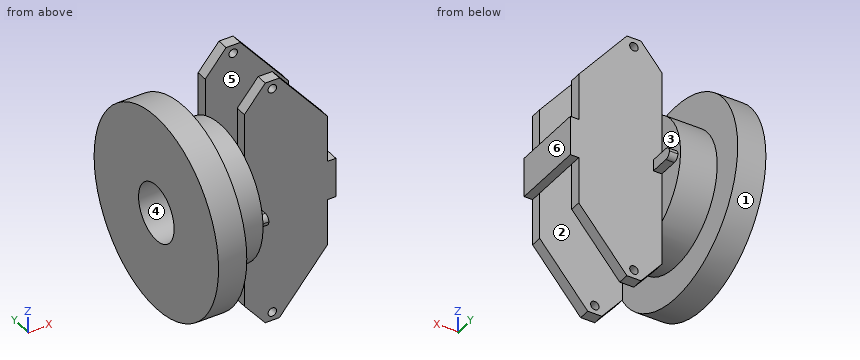
```python
from build123d import *

# Parameters (mm, degrees)
SKETCH1_R               = 35
BOSS_EXTRUDE1_DEPTH     = 10
SKETCH2_R               = 23.5
BOSS_EXTRUDE2_DEPTH     = 13
BOSS_EXTRUDE3_DEPTH     = 4
SKETCH5_R               = 1.5
CUT_EXTRUDE1_DEPTH      = 4
MIRROR3_COPY_1_SKETCH_R = 1.5
MIRROR3_COPY_1_DEPTH    = 4
BOSS_EXTRUDE4_DEPTH     = 3
FILLET1_R               = 2
FILLET1_OF_MIRROR5_R    = 2
SKETCH8_W               = 14
SKETCH8_H               = 26
BOSS_EXTRUDE5_DEPTH     = 3
SKETCH9_R               = 10
CUT_EXTRUDE2_DEPTH      = 10


with BuildPart() as part:
    # Sketch1 → Boss-Extrude1 (new body)
    with BuildSketch(Plane(origin=(0, 0, 0), x_dir=(0, 0, -1), z_dir=(1, 0, 0))):
        Circle(SKETCH1_R)
    extrude(amount=BOSS_EXTRUDE1_DEPTH)

    # Sketch2 → Boss-Extrude2 (add)
    with BuildSketch(Plane(origin=(10, 0, 0), x_dir=(0, 0, -1), z_dir=(1, 0, 0))):
        with Locations(Location((0, 0, 0), (0, 0, 180))):
            Circle(SKETCH2_R)
    extrude(amount=BOSS_EXTRUDE2_DEPTH)

    # Sketch3 → Boss-Extrude3 (add)
    with BuildSketch(Plane(origin=(0, 13, 0), x_dir=(1, 0, 0), z_dir=(0, 1, 0))):
        Polygon((23, 35), (23, -35), (30.392057511, -43.809511096), (35.392057511, -43.809511096), (52.421803319, -23.514250349), (52.421803319, 0), (52.421803319, 23.514250349), (35.392057511, 43.809511096), (30.392057511, 43.809511096), align=None)
    boss_extrude3 = extrude(amount=-BOSS_EXTRUDE3_DEPTH)

    # Sketch5 → Cut-Extrude1 (cut)
    with BuildSketch(Plane(origin=(0, 13, 0), x_dir=(1, 0, 0), z_dir=(0, 1, 0))):
        with Locations(Location((32.892057511, -40.809511096, 0), (0, 0, 270))):
            Circle(SKETCH5_R)
    cut_extrude1 = extrude(amount=-CUT_EXTRUDE1_DEPTH, mode=Mode.SUBTRACT)

    # Mirror2: Cut-Extrude1 across plane
    add(cut_extrude1.mirror(Plane.XY), mode=Mode.SUBTRACT)

    # Mirror3: Boss-Extrude3, Cut-Extrude1 across plane
    add(boss_extrude3.mirror(Plane.ZX))
    add(cut_extrude1.mirror(Plane.ZX), mode=Mode.SUBTRACT)

    # Mirror3 copy 1 sketch → Mirror3 copy 1 (cut)
    with BuildSketch(Plane.XZ.offset(13)):
        with Locations(Location((32.892057511, -40.809511096, 0), (0, 0, 270))):
            Circle(MIRROR3_COPY_1_SKETCH_R)
    extrude(amount=-MIRROR3_COPY_1_DEPTH, mode=Mode.SUBTRACT)

    # Sketch7 → Boss-Extrude4 (add)
    with BuildSketch(Plane(origin=(23, 0, 0), x_dir=(0, 0, -1), z_dir=(1, 0, 0))):
        Polygon((0, 22), (-2, 22), (-2, 13), (2, 13), (2, 22), align=None)
    boss_extrude4 = extrude(amount=BOSS_EXTRUDE4_DEPTH)

    # Fillet1
    fillet1_edges = [part.edges().sort_by_distance(p)[0] for p in [
        (24.5, 22, 2),
        (24.5, 22, -2),
    ]]
    fillet(fillet1_edges, radius=FILLET1_R - 0.0001)  # a hair under: the kernel refuses the full size

    # Mirror5: Boss-Extrude4 across plane
    add(boss_extrude4.mirror(Plane.ZX))

    # Fillet1 of Mirror5
    fillet1_of_mirror5_edges = [part.edges().sort_by_distance(p)[0] for p in [
        (24.5, -22, 2),
        (24.5, -22, -2),
    ]]
    fillet(fillet1_of_mirror5_edges, radius=FILLET1_OF_MIRROR5_R - 0.0001)  # a hair under: the kernel refuses the full size

    # Sketch8 → Boss-Extrude5 (add)
    with BuildSketch(Plane(origin=(52.421803319, 0, 0), x_dir=(0, 0, -1), z_dir=(1, 0, 0))):
        Rectangle(SKETCH8_W, SKETCH8_H)
    extrude(amount=BOSS_EXTRUDE5_DEPTH)

    # Sketch9 → Cut-Extrude2 (cut)
    with BuildSketch(Plane.ZY):
        Circle(SKETCH9_R)
    extrude(amount=-CUT_EXTRUDE2_DEPTH, mode=Mode.SUBTRACT)


solid = part.part
```
Here's how the part is built. I have some questions about the finished solid (model axes, mm). Face numbers are marked on the shaded views. A direction names the side the tool comes from. Coordinates: 2 decimals unless noted, no trailing zeros. Order: outer loops, then holes, each group sorted by start corner. A loop starts at its lowest first (then second) coordinate and runs counter-clockwise, first axis right, second up. Notation, with made-up numbers: (85, -36) -> (89, -36) arc R16 ccw to (89, -18) -> close; hole circle Ø9 at (-8, 23). An arc over 180 degrees is marked (long way). Return JSON: item names as keys, results as strings.
1) I'm going to push flat-ended pins straight in: P1, Ø4.5, axis at y = 11.5, z = 15.5, coming from the +X side; P2, Ø3, axis at x = 41.5, z = -17.5, coming from the +Y side; P3, Ø4.5, axis at y = 10, z = 27.5, coming from the -X side; P4, Ø2.5, axis at x = 24.5, y = 15, coming from the +Z side. Where does each tip first touch, or does it pass through?
Conclusion:
{"P1": "stops at x = 52.42", "P2": "stops at y = 13", "P3": "stops at x = 0", "P4": "stops at z = 2"}
2) On a 3-axis mill with a long thin cutter (end or side, diameter ignored), from which of +Z, -Z, +X, -X, +Y, -Y can I reach the whole of each face in a straight line? I mean the marked faces 4, 5 and 6. Say none if no direction works.
Conclusion:
{"face 4": "-X", "face 5": "+Z, -Z", "face 6": "+Z, -Z, +X, +Y, -Y"}
3) Thinking about a two-plate mould opening in Y: for the marked faces 1, 2 and 3, which applies, +Y half, -Y half, draft (parallel to the pull), parting line (faces both ways), or undercut?
Conclusion:
{"face 1": "parting line", "face 2": "undercut", "face 3": "draft"}
4) If we section it at B-B on x = 41.5: List the corners of the cut face in (y, z) for me.
Conclusion:
{"outline": "(-13, -36.53) -> (-9, -36.53) -> (-9, 36.53) -> (-13, 36.53) -> close; (9, -36.53) -> (13, -36.53) -> (13, 36.53) -> (9, 36.53) -> close"}
5) If we section it at C-C on x = 6.5: List the corners of the cut face in (y, z) for me, plus the area to 3 significant figures.
Conclusion:
{"outline": "circle Ø70 at (0, 0); hole circle Ø20 at (0, 0)", "area": "3,530 mm²"}
6) If we section it at A-A on y = 0: List the corners of the cut face in (x, z) for me, plus the area to 3 significant figures.
Conclusion:
{"outline": "(0, -35) -> (10, -35) -> (10, -23.5) -> (23, -23.5) -> (23, 23.5) -> (10, 23.5) -> (10, 35) -> (0, 35) -> (0, 10) -> (10, 10) -> (10, -10) -> (0, -10) -> close; (52.42, -7) -> (55.42, -7) -> (55.42, 7) -> (52.42, 7) -> close", "area": "1,150 mm²"}
7) If we section it at D-D on y = 7.5: List the corners of the cut face in (x, z) for me, plus the area to 3 significant figures.
Conclusion:
{"outline": "(0, -34.19) -> (10, -34.19) -> (10, -22.27) -> (23, -22.27) -> (23, 22.27) -> (10, 22.27) -> (10, 34.19) -> (0, 34.19) -> (0, 6.61) -> (10, 6.61) -> (10, -6.61) -> (0, -6.61) -> close; (52.42, -7) -> (55.42, -7) -> (55.42, 7) -> (52.42, 7) -> close", "area": "1,170 mm²"}
8) If I drill on probe 1 along Z at (x, y) = (16, -1); probe 2 along X at (y, z) = (0.5, -18.5); probe 3 along Y at (x, z) = (35, -17.5), over which ranges is the centre line in solid material (lowest first)?
Conclusion:
{"probe 1": "z = -23.48 to 23.48", "probe 2": "x = 0 to 23", "probe 3": "y = -13 to -9, 9 to 13"}
